Geometry: final body of the model. Coordinates: model frame, mm. Face numbers are marked on the shaded views. A direction names the side the tool comes from. Give positions to 0.01 mm unless a question says otherwise; leave off trailing zeros. Order: outer loops, then holes, each group sorted by start corner. A loop starts at its lowest first (then second) coordinate and runs counter-clockwise, first axis right, second up. Notation, with made-up numbers: (80, 15.5) - (129, 15.5) arc R30 cw to (129, 40.5) - close; hole circle Ø6 at (-14.75, 4). An arc over 180 degrees is marked (long way). Write item = value, one per line. Start each with the question number.
from build123d import *

# Parameters (mm, degrees)
F0_R     = 12.5
F1_DEPTH = 25
F2_W     = 50
F2_H     = 50
F2_R     = 12.5
F3_DEPTH = 75
F4_R     = 12.5
F5_DEPTH = 50.001


with BuildPart() as f1:
    # F0 (on Front) → F1 (new body)
    with BuildSketch(Plane.XZ):
        Circle(F0_R)
    extrude(amount=F1_DEPTH)

    # F2 (on face) → F3 (join)
    with BuildSketch(Plane.XZ.offset(25)):
        Rectangle(F2_W, F2_H)
        Circle(F2_R, mode=Mode.SUBTRACT)
        Circle(F2_R)
    extrude(amount=F3_DEPTH)

    # F4 (on face) → F5 (cut, through all)
    with BuildSketch(Plane.YZ.offset(25)):
        with Locations((-62.5, 0)):
            Circle(F4_R)
    extrude(amount=-F5_DEPTH, mode=Mode.SUBTRACT)


solid = f1.part
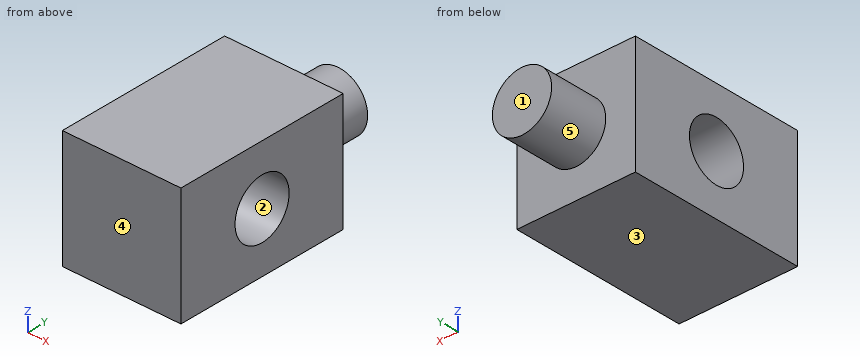
Q1. Section C-C, the plane x = 0. Return the cut outline in (y, z), then the cut area to 3 significant figures.
Q2. Material intervals for line 1 along Z through (x, y) = (4.5, -62.5); line 2 along Y through (x, z) = (-5.5, 10); line 3 along Y through (x, z) = (-10, -16), sorted ascending. Write a range as from..to.
Q3. Section D-D, the plane z = 8. Return the cut outline in (x, y), then the cut area to 3 significant figures.
Q4. Contact query for flat-ended pins moving along their axis: pin 1 (15 mm diameter, centred on y = -62.5, z = 0, fed in from +X); pin 2 (10 mm diameter, centred on y = -14, z = 16, fed in from -X); pin 3 (3 mm diameter, centred on x = 2.5, z = -14, fed in from +Y). Output: stop coordinate, or through.
Q5. Set-up query: the marked faces 4 and 5. Return all of +Z, -Z, +X, -X, +Y, -Y with unobstructed straight access to the full face (end or side cutting, diameter ignored); none if empty.
Q6. Pull-direction query (Y, two-part tool) for the marked faces 1, 2 and 3; classes: +Y half, -Y half, draft (parallel to the pull), parting line (faces both ways), or undercut.
Q7. Section B-B, the plane z = 0. Return the cut outline in (x, y), then the cut area to 4 significant figures.
Q8. Section A-A, the plane y = -62.5. Return the cut outline in (x, z).
The answers:
q1.outline = (-100, -25) - (-25, -25) - (-25, -12.5) - (0, -12.5) - (0, 12.5) - (-25, 12.5) - (-25, 25) - (-100, 25) - close; hole circle Ø25 at (-62.5, 0)
q1.area = 3,880 mm²
q2.line_1 = -25..-12.5, 12.5..25
q2.line_2 = -100..-70, -55..0
q2.line_3 = -100..-25
q3.outline = (-25, -100) - (25, -100) - (25, -72.1) - (-25, -72.1) - close; (-25, -52.9) - (25, -52.9) - (25, -25) - (9.6, -25) - (9.6, 0) - (-9.6, 0) - (-9.6, -25) - (-25, -25) - close
q3.area = 3,270 mm²
q4.pin_1 = through
q4.pin_2 = -5.94
q4.pin_3 = -25
q5.face_4 = +Z, -Z, +X, -X, -Y
q5.face_5 = +Y
q6.face_1 = +Y half
q6.face_2 = undercut
q6.face_3 = draft
q7.outline = (-25, -100) - (25, -100) - (25, -75) - (-25, -75) - close; (-25, -50) - (25, -50) - (25, -25) - (12.5, -25) - (12.5, 0) - (-12.5, 0) - (-12.5, -25) - (-25, -25) - close
q7.area = 3,125 mm²
q8.outline = (-25, -25) - (25, -25) - (25, -12.5) - (-25, -12.5) - close; (-25, 12.5) - (25, 12.5) - (25, 25) - (-25, 25) - close
